from build123d import *

# Parameters (mm, degrees)
SKETCH1_R           = 8.95
BOSS_EXTRUDE1_DEPTH = 6.35


with BuildPart() as part:
    # Sketch1 → Boss-Extrude1 (new body)
    with BuildSketch(Plane.XY):
        with BuildLine():
            Line((0, 0), (34.4805, 0))
            Line((34.4805, 0), (34.4805, 10.16))
            Line((34.4805, 10.16), (32.5755, 10.16))
            Line((32.5755, 10.16), (32.5755, 14.224))
            Line((32.5755, 14.224), (40.4495, 14.224))
            Line((40.4495, 14.224), (40.4495, 10.16))
            Line((40.4495, 10.16), (38.5445, 10.16))
            Line((38.5445, 10.16), (38.5445, 0))
            Line((38.5445, 0), (73.025, 0))
            Line((73.025, 0), (73.025, 101.6))
            Line((73.025, 101.6), (79.375, 101.6))
            Line((79.375, 101.6), (79.375, 0))
            Line((79.375, 0), (110.6805, 0))
            Line((110.6805, 0), (110.6805, 10.16))
            Line((110.6805, 10.16), (108.7755, 10.16))
            Line((108.7755, 10.16), (108.7755, 14.224))
            Line((108.7755, 14.224), (116.6495, 14.224))
            Line((116.6495, 14.224), (116.6495, 10.16))
            Line((116.6495, 10.16), (114.7445, 10.16))
            Line((114.7445, 10.16), (114.7445, 0))
            Line((114.7445, 0), (149.225, 0))
            Line((149.225, 0), (149.225, 152.4))
            Line((149.225, 152.4), (155.575, 152.4))
            Line((155.575, 152.4), (155.575, 0))
            Line((155.575, 0), (186.8805, 0))
            Line((186.8805, 0), (186.8805, 10.16))
            Line((186.8805, 10.16), (184.9755, 10.16))
            Line((184.9755, 10.16), (184.9755, 14.224))
            Line((184.9755, 14.224), (192.8495, 14.224))
            Line((192.8495, 14.224), (192.8495, 10.16))
            Line((192.8495, 10.16), (190.9445, 10.16))
            Line((190.9445, 10.16), (190.9445, 0))
            Line((190.9445, 0), (225.425, 0))
            Line((225.425, 0), (225.425, 101.6))
            Line((225.425, 101.6), (231.775, 101.6))
            Line((231.775, 101.6), (231.775, 0))
            Line((231.775, 0), (263.0805, 0))
            Line((263.0805, 0), (263.0805, 10.16))
            Line((263.0805, 10.16), (261.1755, 10.16))
            Line((261.1755, 10.16), (261.1755, 14.224))
            Line((261.1755, 14.224), (269.0495, 14.224))
            Line((269.0495, 14.224), (269.0495, 10.16))
            Line((269.0495, 10.16), (267.1445, 10.16))
            Line((267.1445, 10.16), (267.1445, 0))
            Line((267.1445, 0), (304.8, 0))
            add(Edge.make_bspline(
                [(304.8, 406.4), (219.863978117, 208.91880682), (304.8, 0)],
                knots=[0, 0, 0, 1, 1, 1], degree=2))
            Line((304.8, 406.4), (279.4, 406.4))
            Line((279.4, 406.4), (279.4, 412.75))
            Line((279.4, 412.75), (254, 412.75))
            Line((254, 412.75), (254, 406.4))
            Line((254, 406.4), (231.775, 406.4))
            Line((231.775, 406.4), (231.775, 330.2))
            Line((231.775, 330.2), (225.425, 330.2))
            Line((225.425, 330.2), (225.425, 406.4))
            Line((225.425, 406.4), (209.9945, 406.4))
            Line((209.9945, 406.4), (209.9945, 396.24))
            Line((209.9945, 396.24), (211.8995, 396.24))
            Line((211.8995, 396.24), (211.8995, 392.176))
            Line((211.8995, 392.176), (204.0255, 392.176))
            Line((204.0255, 392.176), (204.0255, 396.24))
            Line((204.0255, 396.24), (205.9305, 396.24))
            Line((205.9305, 396.24), (205.9305, 406.4))
            Line((205.9305, 406.4), (190.5, 406.4))
            add(Edge.make_bspline(
                [(190.5, 584.2), (152.371549644, 495.523357598), (190.5, 406.4)],
                knots=[0, 0, 0, 1, 1, 1], degree=2))
            Line((190.5, 584.2), (173.014669528, 584.2))
            Line((173.014669528, 584.2), (173.014669528, 574.04))
            Line((173.014669528, 574.04), (174.919669528, 574.04))
            Line((174.919669528, 574.04), (174.919669528, 569.976))
            Line((174.919669528, 569.976), (167.045669528, 569.976))
            Line((167.045669528, 569.976), (167.045669528, 574.04))
            Line((167.045669528, 574.04), (168.950669528, 574.04))
            Line((168.950669528, 574.04), (168.950669528, 584.2))
            Line((168.950669528, 584.2), (155.575, 584.2))
            Line((155.575, 584.2), (155.575, 558.8))
            Line((155.575, 558.8), (149.225, 558.8))
            Line((149.225, 558.8), (149.225, 584.2))
            Line((149.225, 584.2), (135.849330472, 584.2))
            Line((135.849330472, 584.2), (135.849330472, 574.04))
            Line((135.849330472, 574.04), (137.754330472, 574.04))
            Line((137.754330472, 574.04), (137.754330472, 569.976))
            Line((137.754330472, 569.976), (129.880330472, 569.976))
            Line((129.880330472, 569.976), (129.880330472, 574.04))
            Line((129.880330472, 574.04), (131.785330472, 574.04))
            Line((131.785330472, 574.04), (131.785330472, 584.2))
            Line((131.785330472, 584.2), (114.3, 584.2))
            add(Edge.make_bspline(
                [(114.3, 584.2), (152.428450356, 495.523357598), (114.3, 406.4)],
                knots=[0, 0, 0, 1, 1, 1], degree=2))
            Line((114.3, 406.4), (98.8695, 406.4))
            Line((98.8695, 406.4), (98.8695, 396.24))
            Line((98.8695, 396.24), (100.7745, 396.24))
            Line((100.7745, 396.24), (100.7745, 392.176))
            Line((100.7745, 392.176), (92.9005, 392.176))
            Line((92.9005, 392.176), (92.9005, 396.24))
            Line((92.9005, 396.24), (94.8055, 396.24))
            Line((94.8055, 396.24), (94.8055, 406.4))
            Line((94.8055, 406.4), (79.375, 406.4))
            Line((79.375, 406.4), (79.375, 330.2))
            Line((79.375, 330.2), (73.025, 330.2))
            Line((73.025, 330.2), (73.025, 406.4))
            Line((73.025, 406.4), (50.8, 406.4))
            Line((50.8, 406.4), (50.8, 412.75))
            Line((50.8, 412.75), (25.4, 412.75))
            Line((25.4, 412.75), (25.4, 406.4))
            Line((25.4, 406.4), (0, 406.4))
            add(Edge.make_bspline(
                [(0, 406.4), (84.936021883, 208.91880682), (0, 0)],
                knots=[0, 0, 0, 1, 1, 1], degree=2))
        make_face()
        with Locations((152.4, 495.55130888)):
            Circle(SKETCH1_R, mode=Mode.SUBTRACT)
    extrude(amount=BOSS_EXTRUDE1_DEPTH)


solid = part.part
Design review of the part built by this model. Coordinates are the model's own, in mm. Coordinates: 2 decimals unless noted, no trailing zeros. Loops run counter-clockwise (first coordinate to the right, second up) from the corner with the lowest first, then second, coordinate; pieces in that order, holes last.
Item 1: Clearance check with flat-ended pins moving along their axes: pin 1 (1.9 mm diameter, centred on x = 216.5, z = 2.5, fed in from +Y); pin 2 (1.9 mm diameter, centred on y = 580, z = 4, fed in from +X); pin 3 (1.2 mm diameter, centred on y = 12.5, z = 3.5, fed in from +X). State where each tip first meets the part, or that it passes through.
Completed:
pin 1: stops at y = 406.4
pin 2: stops at x = 189.13
pin 3: stops at x = 300.1
Item 2: Wall thickness on L1, parallel to X at y = 333.5, z = 3 (3 decimals); L2, parallel to Y at x = 152.4, z = 2.25; L3, parallel to X at y = 354, z = 2 (3 decimals): over which ranges is each line inside the solid? List them lowest first.
Completed:
L1: x = 25.462 to 73.025, 79.375 to 225.425, 231.775 to 279.338
L2: y = 152.4 to 486.6, 504.5 to 558.8
L3: x = 19.484 to 73.025, 79.375 to 225.425, 231.775 to 285.316
Item 3: Draft analysis for pull direction X (two halves, no side actions). For faces 1 (the flat face through (150, 231, 6.35)), 2 (the cylindrical face through (157.21, 503.1, 3.13)), state which applies: pulls with the +X half, pulls with the -X half, needs draft (parallel to the pull), parting line crosses it, or undercut.
Completed:
face 1: needs draft
face 2: undercut
Item 4: Add section A-A (x = 237.5). Write out the cut boundary in (y, z), and give its area (3 significant figures).
Completed:
outline: (0, 0) - (406.4, 0) - (406.4, 6.35) - (0, 6.35) - close
area: 2,580 mm2
